Can you work these out from the model? Positions are in its coordinate system, mm. A direction names the side the tool comes from. Round coordinates to 2 decimals unless told otherwise and drop trailing zeros. Order: outer loops, then holes, each group sorted by start corner. A loop starts at its lowest first (then second) coordinate and runs counter-clockwise, first axis right, second up. Notation, with made-up numbers: (-16.75, 28) -> (31.25, 28) arc R17 cw to (31.25, 58) -> close; hole circle Ø4 at (-3, 10.25). An arc over 180 degrees is marked (long way). One line per item, written item: value.
```python
from build123d import *

# Parameters (mm, degrees)
SKETCH3_R                                    = 1.25
CUT_EXTRUDE1_DEPTH                           = 53.777836257
SKETCH5_R                                    = 3
SKETCH6_R                                    = 3
CUT_EXTRUDE2_DEPTH                           = 10
BOSS_EXTRUDE1_DEPTH                          = 15
SKETCH9_R                                    = 2.9
CUT_EXTRUDE3_DEPTH                           = 6.5
CSK_FOR_M3_COUNTERSUNK_FLAT_HEAD_SCR_2_COUNT = 2
CSK_FOR_M3_COUNTERSUNK_FLAT_HEAD_SCR_2_PITCH = 26
CSK_FOR_M3_COUNTERSUNK_FLAT_HEAD_SCR_3_COUNT = 2
CSK_FOR_M3_COUNTERSUNK_FLAT_HEAD_SCR_3_PITCH = 36.769552622
CSK_FOR_M3_COUNTERSUNK_FLAT_HEAD_SCR_4_COUNT = 2
CSK_FOR_M3_COUNTERSUNK_FLAT_HEAD_SCR_4_PITCH = 26
BOSS_EXTRUDE2_DEPTH                          = 15


with BuildPart() as part:
    # Sketch2 → Revolve1 (revolve)
    with BuildSketch(Plane.XY, mode=Mode.PRIVATE) as revolve1_sk:
        Polygon((-25, 3), (-25, 0), (-12.5, 0), (-12.5, -4), (-36.5, -4), (-36.5, 11), (-31.5, 11), (-31.5, 3), align=None)
    revolve(revolve1_sk.sketch.rotate(Axis((0, 0, 0), (0, 1, 0)), 270), axis=Axis((0, 0, 0), (0, 1, 0)))

    # Sketch3 → Cut-Extrude1 (cut, through all)
    with BuildSketch(Plane(origin=(0, 0, 0), x_dir=(1, 0, 0), z_dir=(0, 1, 0))):
        with Locations(Location((-13, 13, 0), (0, 0, 270))):
            Circle(SKETCH3_R)
        with Locations(Location((13, 13, 0), (0, 0, 270))):
            Circle(SKETCH3_R)
        with Locations(Location((13, -13, 0), (0, 0, 270))):
            Circle(SKETCH3_R)
        with Locations(Location((-13, -13, 0), (0, 0, 270))):
            Circle(SKETCH3_R)
    extrude(amount=-CUT_EXTRUDE1_DEPTH, mode=Mode.SUBTRACT)

    # Sketch5 → Cut-Revolve1 (revolve, cut)
    with BuildSketch(Plane.XY, mode=Mode.PRIVATE) as cut_revolve1_sk:
        with Locations((31, 7)):
            Circle(SKETCH5_R)
    revolve(cut_revolve1_sk.sketch.rotate(Axis((0, 0, 0), (0, -1, 0)), 270), axis=Axis((0, 0, 0), (0, -1, 0)), mode=Mode.SUBTRACT)

    # Sketch6 → Cut-Extrude2 (cut)
    with BuildSketch(Plane(origin=(0, 7, 0), x_dir=(1, 0, 0), z_dir=(0, 1, 0))):
        with Locations((0, 31)):
            Circle(SKETCH6_R)
    extrude(amount=CUT_EXTRUDE2_DEPTH, mode=Mode.SUBTRACT)

    # Sketch7 → Boss-Extrude1 (add)
    with BuildSketch(Plane(origin=(0, 11, 0), x_dir=(1, 0, 0), z_dir=(0, 1, 0))):
        with BuildLine():
            Line((-36.5, 0), (-36.5, -41.5))
            Line((-36.5, -41.5), (36.5, -41.5))
            Line((36.5, -41.5), (36.5, 0))
            ThreePointArc((36.5, 0), (0, -36.5), (-36.5, 0))
        make_face()
    extrude(amount=-BOSS_EXTRUDE1_DEPTH)

    # Sketch9 → Cut-Extrude3 (cut)
    with BuildSketch(Plane.XY.offset(41.5)):
        with Locations((-27.5, 3.5)):
            Circle(SKETCH9_R)
        with Locations((27.5, 3.5)):
            Circle(SKETCH9_R)
    extrude(amount=-CUT_EXTRUDE3_DEPTH, mode=Mode.SUBTRACT)

    # Sketch11 → CSK for M3 Countersunk Flat Head Screw1 (revolve, cut)
    with BuildSketch(Plane(origin=(13, 0, -13), x_dir=(0, 0, 1), z_dir=(1, 0, 0))):
        Polygon((0, 0), (0, 4), (1.8, 4), (1.8, 1.85), (3.15, 0.5), (3.15, 0), align=None)
    csk_for_m3_countersunk_flat_head_screw1 = revolve(axis=Axis((13, 6.35, -13), (0, -1, 0)), mode=Mode.SUBTRACT)

    # CSK for M3 Countersunk Flat Head Scr 2: CSK for M3 Countersunk Flat Head Screw1 ×2
    with Locations(*[(0, 0, i * CSK_FOR_M3_COUNTERSUNK_FLAT_HEAD_SCR_2_PITCH) for i in range(1, CSK_FOR_M3_COUNTERSUNK_FLAT_HEAD_SCR_2_COUNT)]):
        add(csk_for_m3_countersunk_flat_head_screw1, mode=Mode.SUBTRACT)

    # CSK for M3 Countersunk Flat Head Scr 3: CSK for M3 Countersunk Flat Head Screw1 ×2
    with Locations(*[Vector(-0.7071067811865476, 0, 0.7071067811865476) * (i * CSK_FOR_M3_COUNTERSUNK_FLAT_HEAD_SCR_3_PITCH) for i in range(1, CSK_FOR_M3_COUNTERSUNK_FLAT_HEAD_SCR_3_COUNT)]):
        add(csk_for_m3_countersunk_flat_head_screw1, mode=Mode.SUBTRACT)

    # CSK for M3 Countersunk Flat Head Scr 4: CSK for M3 Countersunk Flat Head Screw1 ×2
    with Locations(*[(-i * CSK_FOR_M3_COUNTERSUNK_FLAT_HEAD_SCR_4_PITCH, 0, 0) for i in range(1, CSK_FOR_M3_COUNTERSUNK_FLAT_HEAD_SCR_4_COUNT)]):
        add(csk_for_m3_countersunk_flat_head_screw1, mode=Mode.SUBTRACT)

    # Sketch12 → Boss-Extrude2 (add)
    with BuildSketch(Plane(origin=(0, 11, 0), x_dir=(1, 0, 0), z_dir=(0, 1, 0))):
        with BuildLine():
            Line((26.5, 36.5), (0, 36.5))
            ThreePointArc((0, 36.5), (25.809397513, 25.809397513), (36.5, 0))
            Line((36.5, 0), (36.5, 26.5))
            Line((36.5, 26.5), (26.5, 36.5))
        make_face()
        with BuildLine():
            Line((-36.5, 26.5), (-36.5, 0))
            ThreePointArc((-36.5, 0), (-25.809397513, 25.809397513), (0, 36.5))
            Line((0, 36.5), (-26.5, 36.5))
            Line((-26.5, 36.5), (-36.5, 26.5))
        make_face()
    extrude(amount=-BOSS_EXTRUDE2_DEPTH)


solid = part.part
```
Q1. We'd pull the mould along Y, two halves only. Please class faces 1 (the face through (-28, 4, 35)), 2 (the face through (-1.34, 10.47, 31.47)), 3 (the face through (8, -4, 11)): released by +Y, released by -Y, zero draft, split by the parting line, or undercut.
Answers below:
face 1: undercut
face 2: zero draft
face 3: released by -Y
Q2. I want a section at C-C on y = 5. List the corners of the cut face in (x, z) for me, plus the area to 3 significant figures.
Answers below:
outline: (-36.5, -26.5) -> (-26.5, -36.5) -> (26.5, -36.5) -> (36.5, -26.5) -> (36.5, 41.5) -> (29.98, 41.5) -> (29.98, 35) -> (25.02, 35) -> (25.02, 41.5) -> (-25.02, 41.5) -> (-25.02, 35) -> (-29.98, 35) -> (-29.98, 41.5) -> (-36.5, 41.5) -> close; hole circle Ø66.47 at (0, 0)
area: 2,060 mm^2
Q3. On a 3-axis mill with a long thin cutter (end or side, diameter ignored), from which of +Z, -Z, +X, -X, +Y, -Y can I reach the whole of each face in a straight line? I mean faces 4 (the face through (0, 10, -34)), 5 (the face through (-24.734, 4.371, 38.296)), 6 (the face through (0, 4, -36.5)). Say none if no direction works.
Answers below:
face 4: +Y
face 5: +Z
face 6: -Z, +X, -X, +Y, -Y
Q4. I want a section at A-A on x = 0. List the corners of the cut face in (y, z) for me, plus the area to 3 significant figures.
Answers below:
outline: (-4, -36.5) -> (11, -36.5) -> (11, -34) -> (7, -34) arc R3 cw to (4.04, -31.5) -> (3, -31.5) -> (3, -25) -> (0, -25) -> (0, -12.5) -> (-4, -12.5) -> close; (-4, 12.5) -> (0, 12.5) -> (0, 25) -> (3, 25) -> (3, 31.5) -> (4.04, 31.5) arc R3 cw to (9.96, 31.5) -> (11, 31.5) -> (11, 41.5) -> (-4, 41.5) -> close
area: 389 mm^2
Q5. I want a section at B-B on z = 0. List the corners of the cut face in (x, y) for me, plus the area to 3 significant figures.
Answers below:
outline: (-36.5, -4) -> (-12.5, -4) -> (-12.5, 0) -> (-25, 0) -> (-25, 3) -> (-31.5, 3) -> (-31.5, 4.04) arc R3 cw to (-31.5, 9.96) -> (-31.5, 11) -> (-36.5, 11) -> close; (12.5, -4) -> (36.5, -4) -> (36.5, 11) -> (31.5, 11) -> (31.5, 9.96) arc R3 cw to (31.5, 4.04) -> (31.5, 3) -> (25, 3) -> (25, 0) -> (12.5, 0) -> close
area: 319 mm^2
Q6. Will these pins go through, and if not, where does the flat tip stop? pin 1 Ø3 at (x, y) = (26.5, 3.5) entering from +Z; pin 2 Ø7 at (x, z) = (13, 13) entering from +Y; pin 3 Ø2 at (x, z) = (13, -13) entering from +Y.
Answers below:
pin 1: z = 35
pin 2: y = 0
pin 3: through
Q7. Please list where these lines run through material, in increasing order: line 1 along Z through (x, y) = (13, -0.25); line 2 along X through (y, z) = (-0.2, -13); line 3 along X through (y, z) = (-2.6, 13).
Answers below:
line 1: -36.5 to -16.15, -9.85 to 9.85, 16.15 to 41.5
line 2: -36.5 to -16.15, -9.85 to 9.85, 16.15 to 36.5
line 3: -36.5 to -14.8, -11.2 to 11.2, 14.8 to 36.5
